```python
from build123d import *

# Parameters (mm, degrees)
SKETCH_1_R          = 4.1
EXTRUDE_1_DEPTH     = 32
SKETCH_3_R          = 1.35
SKETCH_3_W          = 23
SKETCH_3_H          = 12
CUT_EXTRUDE_1_DEPTH = 5
SKETCH_4_R          = 1.6
CUT_EXTRUDE_2_DEPTH = 10
SKETCH_5_R          = 6
EXTRUDE_2_DEPTH     = 2


with BuildPart() as part:
    # 草图1 → 凸台-拉伸1 (new body)
    with BuildSketch(Plane.XY):
        with BuildLine():
            Line((-32.405771928, 8.673637409), (-5.405771928, 8.673637409))
            Line((-5.405771928, 8.673637409), (0.594228072, 8.673637409))
            ThreePointArc((0.594228072, 8.673637409), (3.594228072, -2.522515014), (-4.601924351, 5.673637409))
            Line((-4.601924351, 5.673637409), (-29.405771928, 5.673637409))
            Line((-29.405771928, 5.673637409), (-29.405771928, -6.326362591))
            Line((-29.405771928, -6.326362591), (-32.405771928, -6.326362591))
            Line((-32.405771928, -6.326362591), (-32.405771928, 5.673637409))
            Line((-32.405771928, 5.673637409), (-32.405771928, 8.673637409))
        make_face()
        with Locations((0.594228072, 2.673637409)):
            Circle(SKETCH_1_R, mode=Mode.SUBTRACT)
    extrude(amount=EXTRUDE_1_DEPTH)

    # 草图3 → 切除-拉伸1 (cut)
    with BuildSketch(Plane.ZY.offset(32.405771928)):
        with Locations((29.75, -0.326362591)):
            Circle(SKETCH_3_R)
        with Locations((2.25, -0.326362591)):
            Circle(SKETCH_3_R)
        with Locations((16, -0.326362591)):
            Rectangle(SKETCH_3_W, SKETCH_3_H)
    extrude(amount=-CUT_EXTRUDE_1_DEPTH, mode=Mode.SUBTRACT)

    # 草图4 → 切除-拉伸2 (cut, symmetric)
    with BuildSketch(Plane(origin=(0, 0, 0), x_dir=(1, 0, 0), z_dir=(0, 1, 0))):
        with Locations((0.594228072, -4.365303353)):
            Circle(SKETCH_4_R)
        with Locations((0.594228072, -28.123934877)):
            Circle(SKETCH_4_R)
    extrude(amount=CUT_EXTRUDE_2_DEPTH, both=True, mode=Mode.SUBTRACT)

    # 草图5 → 凸台-拉伸2 (add)
    with BuildSketch(Plane.XY.offset(32)):
        with Locations((0.594228072, 2.673637409)):
            Circle(SKETCH_5_R)
    extrude(amount=EXTRUDE_2_DEPTH)


solid = part.part
```
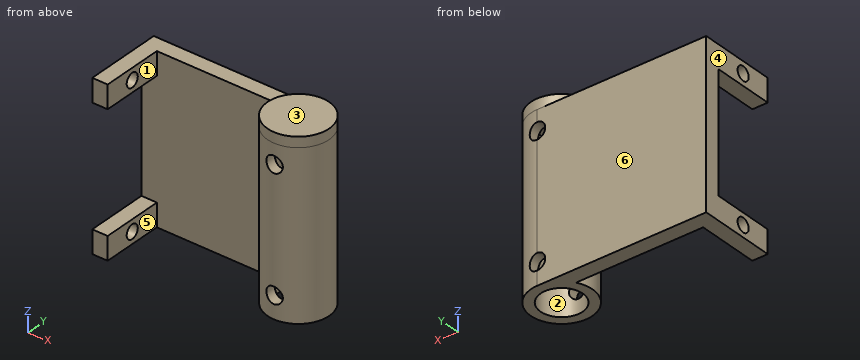
Could you check a few things on this model? Use its own coordinates, in mm. Face numbers are marked on the shaded views. A direction names the side the tool comes from. Round coordinates to 2 decimals unless told otherwise and drop trailing zeros. Write each loop counter-clockwise with the first axis right and the second up, starting at its lowest first coordinate (ties: lowest second). Pieces come first, ordered by that corner, then holes. Notation, with made-up numbers: M 74.25,89.5 L 102.25,89.5 A31 ccw 102.25,121.5 Z; hole C 26,25 d1. An arc over 180 degrees is marked long. Write each question's results on one line, items separated by ' | '. Start each with the question number.
1. Thinking about a two-plate mould opening in X: for the marked faces 4, 5 and 6, which applies, +X half, -X half, draft (parallel to the pull), parting line (faces both ways), or undercut?
2. Imagine slicing it at C-C on x = -0.5. List the corners of the cut face in (y, z) for me.
3. On a 3-axis mill with a long thin cutter (end or side, diameter ignored), from which of +Z, -Z, +X, -X, +Y, -Y can I reach the whole of each face in a straight line? I mean the marked faces 1, 2 and 3. Say none if no direction works.
4. Imagine slicing it at A-A on z = 2. List the corners of the cut face in (x, y) for me, and give its area (3 significant figures).
5. I'm going to push flat-ended pins straight in: pin 1 Ø3 at (x, z) = (0.59, 28.12) entering from +Y; pin 2 Ø5 at (x, z) = (0.59, 4.37) entering from -Y; pin 3 Ø4.5 at (y, z) = (-0.33, 2.25) entering from -X; pin 4 Ø8 at (x, z) = (-9.5, 14) entering from -Y. Where does each tip first touch, or does it pass through?
6. Imagine slicing it at B-B on y = 0.5. List the corners of the cut face in (x, z) for me, and give its area (3 significant figures).
7. I need wall thicknesses on L1, parallel to X at y = 2.75, z = 22.5; L2, parallel to X at y = 3.25, z = 31; L3, parallel to Y at x = -29.5, z = 24.5. Which ranges of each line are inside material? Lowest first, please. Write a range as from..to.
8. Imagine slicing it at D-D on z = 29. List the corners of the cut face in (x, y) for me.
Result sheet:
1) face 4: -X half | face 5: undercut | face 6: draft
2) outline: M -3.23,0 L -1.28,0 L -1.28,3.2 L -3.23,3.2 Z; M -3.23,5.53 L -1.28,5.53 L -1.28,26.96 L -3.23,26.96 Z; M -3.23,29.29 L -1.28,29.29 L -1.28,32 L 6.62,32 L 6.62,29.29 L 8.67,29.29 L 8.67,32 L 8.57,32 L 8.57,34 L -3.23,34 Z; M 6.62,0 L 8.67,0 L 8.67,3.2 L 6.62,3.2 Z; M 6.62,5.53 L 8.67,5.53 L 8.67,26.96 L 6.62,26.96 Z
3) face 1: +Z, -Z, -Y | face 2: -Z | face 3: +Z, +X, -X, +Y, -Y
4) outline: M -32.41,-6.33 L -29.41,-6.33 L -29.41,-1.65 L -32.41,-1.65 Z; M -32.41,1 L -29.41,1 L -29.41,5.67 L -4.6,5.67 A6 ccw long 0.59,8.67 L -32.41,8.67 Z; hole C 0.59,2.67 d8.2 | area: 176 mm^2
5) pin 1: passes through | pin 2: stops at y = -3.33 | pin 3: stops at x = -32.41 | pin 4: stops at y = 5.67
6) outline: M -32.41,0 L -29.41,0 L -29.41,1.18 L -32.41,1.18 Z; M -32.41,3.32 L -29.41,3.32 L -29.41,4.5 L -32.41,4.5 Z; M -32.41,27.5 L -29.41,27.5 L -29.41,28.68 L -32.41,28.68 Z; M -32.41,30.82 L -29.41,30.82 L -29.41,32 L -32.41,32 Z; M -5,0 L -2.88,0 L -2.88,32 L 4.07,32 L 4.07,0 L 6.19,0 L 6.19,34 L -5,34 Z | area: 172 mm^2
7) L1: x = -5.41..-3.51, 4.69..6.59 | L2: x = -32.41..-29.41, -5.38..-3.47, 4.65..6.57 | L3: y = 5.67..8.67
8) outline: M -32.41,-6.33 L -29.41,-6.33 L -29.41,-1.45 L -32.41,-1.45 Z; M -32.41,0.8 L -29.41,0.8 L -29.41,5.67 L -4.6,5.67 A6 ccw -0.74,-3.18 L -0.74,-1.2 A4.1 cw -0.74,6.55 L -0.74,8.67 L -32.41,8.67 Z; M 1.93,-3.18 A6 ccw 1.93,8.52 L 1.93,6.55 A4.1 cw 1.93,-1.2 Z
